from build123d import *

# Parameters (mm, degrees)
FURO_COM_FOLGA_DE_M51_D     = 5.8
FURO_COM_FOLGA_DE_M51_DEPTH = 6
FURO_COM_FOLGA_DE_M51_TIP   = 1.171676055
DOMO1_FACE_RADIUS           = 5
DOMO1_HEIGHT                = 0.5


with BuildPart() as part:
    # Sketch2 → Revolve1 (revolve)
    with BuildSketch(Plane.XY):
        Polygon((-10, 0), (-10, 5), (-9, 5), (-9, 4), (5, 4), (5, 0), align=None)
    revolve(axis=Axis((-33.61911958, 0, 0), (1, 0, 0)))

    # Furo com folga de M51
    with Locations(Plane(origin=(5, 0, 0), x_dir=(0, 0, -1), z_dir=(1, 0, 0))):
        with Locations((0, 0)):
            Hole(FURO_COM_FOLGA_DE_M51_D / 2, depth=FURO_COM_FOLGA_DE_M51_DEPTH)
            with Locations((0, 0, -(FURO_COM_FOLGA_DE_M51_DEPTH + FURO_COM_FOLGA_DE_M51_TIP / 2))):  # 136° drill point
                Cone(0, FURO_COM_FOLGA_DE_M51_D / 2, FURO_COM_FOLGA_DE_M51_TIP, mode=Mode.SUBTRACT)

    # Domo1: a dome of height H over a round flat face of radius A is a cap of a sphere of radius (A * A + H * H) / (2 * H)
    domo1_r = (DOMO1_FACE_RADIUS * DOMO1_FACE_RADIUS + DOMO1_HEIGHT * DOMO1_HEIGHT) / (2 * DOMO1_HEIGHT)
    domo1_base = Plane((-10, 0, 0), z_dir=(-1, 0, 0))
    with Locations(domo1_base.offset(DOMO1_HEIGHT - domo1_r)):
        domo1_ball = Sphere(domo1_r, mode=Mode.PRIVATE)
    add(split(domo1_ball, bisect_by=domo1_base, keep=Keep.TOP, mode=Mode.PRIVATE))


solid = part.part
Can you work these out from the model? Positions are in its coordinate system, mm. A direction names the side the tool comes from. Round coordinates to 2 decimals unless told otherwise and drop trailing zeros. Write each loop counter-clockwise with the first axis right and the second up, starting at its lowest first coordinate (ties: lowest second). Pieces come first, ordered by that corner, then holes. Notation, with made-up numbers: (42, 60.25) - (86, 60.25) arc R15 cw to (86, 83.25) - close; hole circle Ø1 at (75.5, -30). An arc over 180 degrees is marked (long way). Write each question's results on one line, items separated by ' | '. Start each with the question number.
1) Which directions (+Z, -Z, +X, -X, +Y, -Y) give clear straight access to the entire face, cutting with the end or side of a thin tool? Please do faces 4 (the cylindrical face through (-9.49, -1.08, -4.88)), 5 (the cylindrical face through (2, 0.1, -2.9)).
2) Suppose I cut it at B-B (y = 3.25). List the corners of the cut face in (x, z) for me.
3) Suppose I cut it at C-C (x = 1). List the corners of the cut face in (y, z) for me, and give its area (3 significant figures).
4) Suppose I cut it at A-A (x = -3.25). List the corners of the cut face in (y, z) for me, and give its area (3 significant figures).
5) For pin 1 Ø6 at (x, y) = (-5, 2) entering from +Z; pin 2 Ø2 at (y, z) = (1, 2.5) entering from -X; pin 3 Ø6 at (x, z) = (0, -3.5) entering from -Y, each with a flat end and sliding along its axis, tell me the tip position at first contact or that it passes through.
6) Please list where these lines run through material, in increasing order: line 1 (Z direction, x = 3.1, y = 0); line 2 (Y direction, x = 0, z = -1.5); line 3 (Y direction, x = -3.75, z = -1.5).
7) We'd pull the mould along Y, two halves only. Please class faces 1 (the cylindrical face through (-1.902, -0.867, -3.905)), 2 (the conical face through (-2.098, -0.069, -0.168)), 3 (the flat face through (5, 3, 1)): released by +Y, released by -Y, zero draft, split by the parting line, or undercut.
Here are the results:
1) face 4: +X, -X | face 5: +X
2) outline: (-10, -3.8) - (-9, -3.8) - (-9, -2.33) - (5, -2.33) - (5, 2.33) - (-9, 2.33) - (-9, 3.8) - (-10, 3.8) arc R25.04 ccw to start
3) outline: circle Ø8 at (0, 0); hole circle Ø5.8 at (0, 0) | area: 23.8 mm2
4) outline: circle Ø8 at (0, 0) | area: 50.3 mm2
5) pin 1: stops at z = 4 | pin 2: stops at x = -10.44 | pin 3: stops at y = -3.97
6) line 1: z = -4 to -2.9, 2.9 to 4 | line 2: y = -3.71 to -2.48, 2.48 to 3.71 | line 3: y = -3.71 to 3.71
7) face 1: split by the parting line | face 2: undercut | face 3: zero draft
